from build123d import *

# Parameters (mm, degrees)
F0_W     = 92
F0_H     = 30
F0_W_2   = 17
F0_H_2   = 22
F1_DEPTH = 30
F2_R     = 5
F3_R     = 2
F4_R     = 1
F5_W     = 1.5
F5_H     = 2
F6_DEPTH = 2
F7_SIZE  = 1
F8_W     = 40
F8_H     = 15
F8_R     = 2.5
F9_DEPTH = 5
F10_R    = 3
F11_SIZE = 0.5


with BuildPart() as f1:
    # F0 (on Top) → F1 (new body)
    with BuildSketch(Plane.XY):
        with Locations((-18.263159, 15)):
            Rectangle(F0_W, F0_H)
        with Locations((-49.763159, 15)):
            Rectangle(F0_W_2, F0_H_2, mode=Mode.SUBTRACT)
        with Locations((-28.763159, 15)):
            Rectangle(F0_W_2, F0_H_2, mode=Mode.SUBTRACT)
        with Locations((-7.763159, 15)):
            Rectangle(F0_W_2, F0_H_2, mode=Mode.SUBTRACT)
        with Locations((13.236841, 15)):
            Rectangle(F0_W_2, F0_H_2, mode=Mode.SUBTRACT)
    extrude(amount=F1_DEPTH)

    # F2
    f2_edges = [f1.edges().sort_by_distance(p)[0] for p in [
        (27.736841, 0, 15),
        (27.736841, 30, 15),
        (-64.263159, 0, 15),
        (-64.263159, 30, 15),
    ]]
    fillet(f2_edges, radius=F2_R)

    # F3
    f3_edges = [f1.edges().sort_by_distance(p)[0] for p in [
        (-18.263159, 0, 30),
        (-18.263159, 30, 30),
    ]]
    fillet(f3_edges, radius=F3_R)

    # F4
    f4_edges = [f1.edges().sort_by_distance(p)[0] for p in [
        (-58.263159, 15, 30),
        (-49.763159, 4, 30),
        (-41.263159, 15, 30),
        (-49.763159, 26, 30),
        (-37.263159, 15, 30),
        (-28.763159, 26, 30),
        (-20.263159, 15, 30),
        (-28.763159, 4, 30),
        (-16.263159, 15, 30),
        (-7.763159, 26, 30),
        (0.736841, 15, 30),
        (-7.763159, 4, 30),
        (4.736841, 15, 30),
        (13.236841, 26, 30),
        (21.736841, 15, 30),
        (13.236841, 4, 30),
    ]]
    fillet(f4_edges, radius=F4_R)

    # F5 (on face) → F6 (join)
    with BuildSketch(Plane(origin=(0, 0, 0), x_dir=(1, 0, 0), z_dir=(0, 0, -1))):
        with Locations((-57.513159, -15)):
            Rectangle(F5_W, F5_H)
        with Locations((-36.513159, -15)):
            Rectangle(F5_W, F5_H)
        with Locations((-15.513159, -15)):
            Rectangle(F5_W, F5_H)
        with Locations((5.486841, -15)):
            Rectangle(F5_W, F5_H)
    extrude(amount=-F6_DEPTH)

    # F7
    f7_edges = [f1.edges().sort_by_distance(p)[0] for p in [
        (-56.763159, 15, 0),
        (-35.763159, 15, 0),
        (-14.763159, 15, 0),
        (6.236841, 15, 0),
    ]]
    chamfer(f7_edges, length=F7_SIZE)

    # F8 (on face) → F9 (join)
    with BuildSketch(Plane(origin=(0, 0, 0), x_dir=(1, 0, 0), z_dir=(0, 0, -1))):
        with Locations((-18.263159, 7.5)):
            Rectangle(F8_W, F8_H)
        with Locations((-30.763159, 7.5)):
            Circle(F8_R, mode=Mode.SUBTRACT)
        with Locations((-5.763159, 7.5)):
            Circle(F8_R, mode=Mode.SUBTRACT)
        Polygon((-59.263159, 0), (-38.263159, 0), (-38.263159, 15), align=None)
        Polygon((1.736841, 15), (1.736841, 0), (22.736841, 0), align=None)
        with Locations((-18.263159, -37.5)):
            Rectangle(F8_W, F8_H)
        with Locations((-30.763159, -37.5)):
            Circle(F8_R, mode=Mode.SUBTRACT)
        with Locations((-5.763159, -37.5)):
            Circle(F8_R, mode=Mode.SUBTRACT)
        Polygon((22.736841, -30), (1.736841, -30), (1.736841, -45), align=None)
        Polygon((-38.263159, -45), (-38.263159, -30), (-59.263159, -30), align=None)
    extrude(amount=-F9_DEPTH)

    # F10
    f10_edges = [f1.edges().sort_by_distance(p)[0] for p in [
        (12.236841, -7.5, 5),
        (-18.263159, -15, 5),
        (-48.763159, -7.5, 5),
        (12.236841, 37.5, 5),
        (-18.263159, 45, 5),
        (-48.763159, 37.5, 5),
    ]]
    fillet(f10_edges, radius=F10_R)

    # F11
    f11_edges = [f1.edges().sort_by_distance(p)[0] for p in [
        (-8.263159, 37.5, 5),
        (-33.263159, 37.5, 5),
        (-8.263159, -7.5, 5),
        (-33.263159, -7.5, 5),
    ]]
    chamfer(f11_edges, length=F11_SIZE)


solid = f1.part
CAD build for the part. Positions are in the model's coordinates, mm. A direction names the side the tool comes from. Give positions to 0.01 mm unless a question says otherwise; leave off trailing zeros. Write each loop counter-clockwise with the first axis right and the second up, starting at its lowest first coordinate (ties: lowest second). Pieces come first, ordered by that corner, then holes. Notation, with made-up numbers: (-24.5, 27.25) -> (15.5, 27.25) arc R22 cw to (15.5, 50.25) -> close; hole circle Ø2 at (1.5, 49). An arc over 180 degrees is marked (long way). Return JSON: item names as keys, results as strings.
Item 1: Drill centre lines: probe 1 along X at (y, z) = (8.5, 4.5); probe 2 along Y at (x, z) = (-34, 15); probe 3 along X at (y, z) = (-7, 1). Where is each one in solid material? Low to high.
Answer below:
{"probe 1": "x = -64.26 to -58.26, -41.26 to -37.26, -20.26 to -16.26, 0.74 to 4.74, 21.74 to 27.74", "probe 2": "y = 0 to 4, 26 to 30", "probe 3": "x = -49.46 to -33.21, -28.31 to -8.21, -3.31 to 12.94"}
Item 2: Band-saw the part on A-A (y = 6). Give the number of separate pieces and of enclosed holes in the cut face, then the cut area to 3 significant figures.
Answer below:
{"separate pieces": "5", "enclosed holes": "0", "area": "717 mm2"}
Item 3: Band-saw the part on B-B (x = -12.5). List the corners of the cut face in (y, z), then the cut area to 3 significant figures.
Answer below:
{"outline": "(-15, 0) -> (4, 0) -> (4, 29) arc R1 ccw to (3, 30) -> (2, 30) arc R2 ccw to (0, 28) -> (0, 5) -> (-12, 5) arc R3 ccw to (-15, 2) -> close; (26, 0) -> (45, 0) -> (45, 2) arc R3 ccw to (42, 5) -> (30, 5) -> (30, 28) arc R2 ccw to (28, 30) -> (27, 30) arc R1 ccw to (26, 29) -> close", "area": "384 mm2"}
Item 4: Tool access for faces 1 (the flat face through (-19, -5, 5)), 2 (the flat face through (-19, 15, 0)), 3 (the flat face through (-29, 26, 14)): list every direction of +Z, -Z, +X, -X, +Y, -Y with a clear straight run to the whole face (end or side of a thin tool).
Answer below:
{"face 1": "+Z, +X, -X, -Y", "face 2": "-Z, +X, -X, +Y, -Y", "face 3": "+Z, -Z"}
Item 5: Band-saw the part on C-C (z = 24). List the corners of the cut face in (x, y).
Answer below:
{"outline": "(-64.26, 5) arc R5 ccw to (-59.26, 0) -> (22.74, 0) arc R5 ccw to (27.74, 5) -> (27.74, 25) arc R5 ccw to (22.74, 30) -> (-59.26, 30) arc R5 ccw to (-64.26, 25) -> close; hole (-58.26, 4) -> (-41.26, 4) -> (-41.26, 26) -> (-58.26, 26) -> close; hole (-37.26, 4) -> (-20.26, 4) -> (-20.26, 26) -> (-37.26, 26) -> close; hole (-16.26, 4) -> (0.74, 4) -> (0.74, 26) -> (-16.26, 26) -> close; hole (4.74, 4) -> (21.74, 4) -> (21.74, 26) -> (4.74, 26) -> close"}
Item 6: Two-plate mould, pull along Y, no slides. Class faces 4 (the cylindrical face through (27.135, 15.14, 29.43)), 5 (the cylindrical face through (-48.119, 36.909, 4.098)), 6 (the flat face through (-50, 4, 14)): +Y half, -Y half, draft (parallel to the pull), parting line (faces both ways), or undercut.
Answer below:
{"face 4": "draft", "face 5": "+Y half", "face 6": "undercut"}
Item 7: Drop flat-ended pins along their axis: pin 1 (6 mm diameter, centred on y = 30, z = 5, fed in from -X); pin 2 (8 mm diameter, centred on x = -10.5, z = 14.5, fed in from -Y); pin 3 (3 mm diameter, centred on x = -45.5, z = 11.5, fed in from +Y); pin 4 (4 mm diameter, centred on x = -5.76, y = 37.5, fed in from +Z). Give the stop position or say it passes through.
Answer below:
{"pin 1": "stops at x = -63.85", "pin 2": "stops at y = 0", "pin 3": "stops at y = 30", "pin 4": "passes through"}
